from build123d import *

# Parameters (mm, degrees)
FILLET1_R           = 2.159
SKETCH6_R           = 2.0828
BOSS_EXTRUDE1_DEPTH = 21.59
CHAMFER2_SIZE       = 0.635


with BuildPart() as part:
    # Sketch1 → Revolve1 (revolve)
    with BuildSketch(Plane.XY, mode=Mode.PRIVATE) as revolve1_sk:
        Polygon((31.75, 0), (31.75, 4.28625), (11.64625, 4.28625), (10.16, 2.8), (0, 2.8), (0, 0), align=None)
    revolve(revolve1_sk.sketch.rotate(Axis((0, 0, 0), (1, 0, 0)), 90), axis=Axis((0, 0, 0), (1, 0, 0)))

    # Fillet1
    fillet1_edges = [part.edges().sort_by_distance(p)[0] for p in [
        (11.64625, 0, -4.28625),
    ]]
    fillet(fillet1_edges, radius=FILLET1_R)

    # Sketch6 → Boss-Extrude1 (add)
    with BuildSketch(Plane.ZY):
        Circle(SKETCH6_R)
    extrude(amount=BOSS_EXTRUDE1_DEPTH)

    # Chamfer2
    chamfer2_edges = [part.edges().sort_by_distance(p)[0] for p in [
        (-21.59, 0, -2.0828),
    ]]
    chamfer(chamfer2_edges, length=CHAMFER2_SIZE)


solid = part.part
Design review of the part built by this model. Coordinates are the model's own, in mm. A direction names the side the tool comes from. Round coordinates to 2 decimals unless told otherwise and drop trailing zeros. Write each loop counter-clockwise with the first axis right and the second up, starting at its lowest first coordinate (ties: lowest second). Pieces come first, ordered by that corner, then holes.
Item 1: For pin 1 Ø5 at (x, z) = (4, 2.5) entering from -Y, flat-tipped, find the tip position at first contact; note if it passes through.
Item 2: Wall thickness on L1, parallel to X at y = 1.25, z = -2; L2, parallel to Z at x = 18, y = 0.25; L3, parallel to Y at x = -1.5, z = 0: over which ranges is each line inside the solid? List them lowest first.
Item 3: Consider section B-B on x = -13.5. Give the boundary of the cut face in (y, z).
Item 4: Consider section A-A on x = 7. Give the boundary of the cut face in (y, z).
Item 5: For faces 1 (the flat face through (31.75, 0, 0)), 2 (the flat face through (0, 1, -2)), list the 3-axis set-ups (+Z, -Z, +X, -X, +Y, -Y) from which the entire face can be reached by the end or side of a thin tool; tool diameter is ignored.
Check values:
1. pin 1: stops at y = -2.8
2. L1: x = 0 to 31.75
2. L2: z = -4.28 to 4.28
2. L3: y = -2.08 to 2.08
3. outline: circle Ø4.17 at (0, 0)
4. outline: circle Ø5.6 at (0, 0)
5. face 1: +Z, -Z, +X, +Y, -Y
5. face 2: -X
